```python
from build123d import *

# Parameters (mm, degrees)
BOSS_EXTRUDE1_DEPTH = 2
BOSS_EXTRUDE2_DEPTH = 2
BOSS_EXTRUDE3_DEPTH = 2
CUT_EXTRUDE1_REACH  = 192.961
FILLET1_R           = 0.5
CUT_EXTRUDE3_REACH  = 192.929
SKETCH4_R           = 1.4
CUT_EXTRUDE4_REACH  = 192.929
SKETCH9_R           = 0.5


with BuildPart() as part:
    # Sketch2 → Boss-Extrude1 (new body)
    with BuildSketch(Plane.XY):
        with BuildLine():
            Line((0, 135), (0, 110))
            ThreePointArc((0, 110), (77.781745931, 77.781745931), (110, 0))
            Line((110, 0), (135, 0))
            ThreePointArc((135, 0), (95.45941546, 95.45941546), (0, 135))
        make_face()
    extrude(amount=BOSS_EXTRUDE1_DEPTH)

    # Sketch3 → Boss-Extrude2 (add)
    with BuildSketch(Plane(origin=(0, 0, 0), x_dir=(-1, 0, 0), z_dir=(0, 0, -1))):
        with BuildLine():
            Line((0, 125.8), (0, 125))
            ThreePointArc((0, 125), (-88.388347648, 88.388347648), (-125, 0))
            Line((-125, 0), (-125.8, 0))
            ThreePointArc((-125.8, 0), (-88.954033073, 88.954033073), (0, 125.8))
        make_face()
    extrude(amount=BOSS_EXTRUDE2_DEPTH)

    # Sketch7 → Boss-Extrude3 (add)
    with BuildSketch(Plane.XY):
        Polygon((114.100254777, 0), (120.899745223, 0), (121.392602365, -6.9), (113.607397635, -6.9), align=None)
    extrude(amount=BOSS_EXTRUDE3_DEPTH)

    # Sketch8 → Cut-Extrude1 (cut, up to next)
    with BuildSketch(Plane.XY.offset(2), mode=Mode.PRIVATE) as cut_extrude1_sk1:
        Polygon((-0.007124705, 121.09974587), (-0.007124705, 113.90025413), (7.1, 113.392602365), (7.1, 121.607397635), align=None)
    cut_extrude1_tool1 = extrude(cut_extrude1_sk1.sketch, amount=-CUT_EXTRUDE1_REACH, mode=Mode.PRIVATE) & part.part
    add(cut_extrude1_tool1.solids().sort_by_distance((3.624459, 117.5, 2))[0], mode=Mode.SUBTRACT)

    # Fillet1
    fillet1_edges = [part.edges().sort_by_distance(p)[0] for p in [
        (120.899745223, 0, 1),
        (121.392602365, -6.9, 1),
        (113.607397635, -6.9, 1),
        (114.100254777, 0, 1),
        (0, 113.899745223, 1),
        (0, 121.100254777, 1),
        (7.1, 113.392602365, 1),
        (7.1, 121.607397635, 1),
    ]]
    fillet(fillet1_edges, radius=FILLET1_R)

    # Sketch4 → Cut-Extrude3 (cut, up to next)
    with BuildSketch(Plane.XY, mode=Mode.PRIVATE) as cut_extrude3_sk1:
        with Locations(Location((58.75, 101.757984945, 0), (0, 0, 180))):
            Circle(SKETCH4_R)
    cut_extrude3_tool1 = extrude(cut_extrude3_sk1.sketch, amount=CUT_EXTRUDE3_REACH, mode=Mode.PRIVATE) & part.part
    # Sketch4 → Cut-Extrude3 (cut, up to next)
    with BuildSketch(Plane.XY, mode=Mode.PRIVATE) as cut_extrude3_sk2:
        with Locations(Location((101.757984945, 58.75, 0), (0, 0, 180))):
            Circle(SKETCH4_R)
    cut_extrude3_tool2 = extrude(cut_extrude3_sk2.sketch, amount=CUT_EXTRUDE3_REACH, mode=Mode.PRIVATE) & part.part
    # Sketch4 → Cut-Extrude3 (cut, up to next)
    with BuildSketch(Plane.XY, mode=Mode.PRIVATE) as cut_extrude3_sk3:
        with Locations(Location((117.5, 0, 0), (0, 0, 180))):
            Circle(SKETCH4_R)
    cut_extrude3_tool3 = extrude(cut_extrude3_sk3.sketch, amount=CUT_EXTRUDE3_REACH, mode=Mode.PRIVATE) & part.part
    add(cut_extrude3_tool1.solids().sort_by_distance((58.75, 101.757985, 0))[0], mode=Mode.SUBTRACT)
    add(cut_extrude3_tool2.solids().sort_by_distance((101.757985, 58.75, 0))[0], mode=Mode.SUBTRACT)
    add(cut_extrude3_tool3.solids().sort_by_distance((117.5, 0, 0))[0], mode=Mode.SUBTRACT)

    # Sketch9 → Cut-Extrude4 (cut, up to next)
    with BuildSketch(Plane(origin=(0, 0, 0), x_dir=(-1, 0, 0), z_dir=(0, 0, -1)), mode=Mode.PRIVATE) as cut_extrude4_sk1:
        with Locations((-93.268471003, 86.197403191)):
            Circle(SKETCH9_R)
    cut_extrude4_tool1 = extrude(cut_extrude4_sk1.sketch, amount=-CUT_EXTRUDE4_REACH, mode=Mode.PRIVATE) & part.part
    # Sketch9 → Cut-Extrude4 (cut, up to next)
    with BuildSketch(Plane(origin=(0, 0, 0), x_dir=(-1, 0, 0), z_dir=(0, 0, -1)), mode=Mode.PRIVATE) as cut_extrude4_sk2:
        with Locations((-86.197403191, 93.268471003)):
            Circle(SKETCH9_R)
    cut_extrude4_tool2 = extrude(cut_extrude4_sk2.sketch, amount=-CUT_EXTRUDE4_REACH, mode=Mode.PRIVATE) & part.part
    add(cut_extrude4_tool1.solids().sort_by_distance((93.268471, 86.197403, 0))[0], mode=Mode.SUBTRACT)
    add(cut_extrude4_tool2.solids().sort_by_distance((86.197403, 93.268471, 0))[0], mode=Mode.SUBTRACT)


solid = part.part
```
CAD build for the part. Positions are in the model's coordinates, mm. A direction names the side the tool comes from. Give positions to 0.01 mm unless a question says otherwise; leave off trailing zeros. Order: outer loops, then holes, each group sorted by start corner. A loop starts at its lowest first (then second) coordinate and runs counter-clockwise, first axis right, second up.
(1) Saw through at B-B, the plane z = 0.7. Give the cut face in (x, y), then the cut area to 3 significant figures.
(2) Drill centre lines: L1, parallel to Z at x = 11, y = 125.5; L2, parallel to X at y = 58.75, z = 1.45; L3, parallel to Y at x = 52.5, z = -1. Where is each one in solid material? Low to high.
(3) Tool access for faces 1 (the flat face through (71.5, 83.8, 0)), 2 (the flat face through (128, 0, 1)), 3 (the flat face through (92, 88, 0)): list every direction of +Z, -Z, +X, -X, +Y, -Y with a clear straight run to the whole face (end or side of a thin tool).
(4) Saw through at C-C, the plane y = 98.5. Give the cut face in (x, z), then the cut area to 3 significant figures.
(5) Saw through at A-A, the plane x = 19. Give the cut face in (y, z), then the cut area to 3 significant figures.
(6) Flat gauge pins, fed straight in: pin 1 (1.6 mm diameter, centred on y = 116.5, z = 1.5, fed in from -X); pin 2 (1 mm diameter, centred on x = 111.5, z = 1, fed in from -Y). Where does each tip first touch, or does it go through?
Results found:
1. outline: (0, 110) arc R110 cw to (110, 0) - (113.56, 0) arc R0.5 cw to (114.06, -0.54) - (113.65, -6.36) arc R0.5 ccw to (114.14, -6.9) - (120.86, -6.9) arc R0.5 ccw to (121.35, -6.36) - (120.94, -0.54) arc R0.5 cw to (121.44, 0) - (135, 0) arc R135 ccw to (0, 135) - (0, 121.64) arc R0.5 ccw to (0.54, 121.14) - (6.56, 121.57) arc R0.5 cw to (7.1, 121.07) - (7.1, 113.93) arc R0.5 cw to (6.56, 113.43) - (0.54, 113.86) arc R0.5 ccw to (0, 113.36) - close; hole circle Ø2.8 at (58.75, 101.76); hole circle Ø1 at (86.2, 93.27); hole circle Ø1 at (93.27, 86.2); hole circle Ø2.8 at (101.76, 58.75); hole circle Ø2.8 at (117.5, 0)
1. area: 4,790 mm2
2. L1: z = 0 to 2
2. L2: x = 93 to 100.36, 103.16 to 121.55
2. L3: y = 113.44 to 114.32
3. face 1: -Z, -X, -Y
3. face 2: +Z, -Z, +X, -Y
3. face 3: -Z, +X, +Y
4. outline: (48.97, 0) - (76.96, 0) - (76.96, -2) - (78.25, -2) - (78.25, 0) - (92.32, 0) - (92.32, 2) - (48.97, 2) - close
4. area: 89.3 mm2
5. outline: (108.35, 0) - (123.55, 0) - (123.55, -2) - (124.36, -2) - (124.36, 0) - (133.66, 0) - (133.66, 2) - (108.35, 2) - close
5. area: 52.2 mm2
6. pin 1: stops at x = 7.1
6. pin 2: stops at y = 0
